Autodesk Inventor part; units mm, degrees
ref_plane "YZ Plane" through (0, 0, 0) normal (1, 0, 0) x (0, 1, 0)
ref_plane "XZ Plane" through (0, 0, 0) normal (0, 1, 0) x (-1, 0, 0)
ref_plane "XY Plane" through (0, 0, 0) normal (0, 0, 1) x (1, 0, 0)
sketch "Sketch1" plane through (0, 0, 0) normal (0, 1, 0) x (-1, 0, 0)
  line L0 (219, 0) -> (266.75, 0)
  line L1 (266.75, 0) -> (266.75, 2)
  line L2 (266.75, 2) -> (317.5, 2)
  line L3 (317.5, 2) -> (317.5, 40)
  line L4 (317.5, 40) -> (219, 40)
  line L5 (219, 40) -> (219, 0)
  line L6 (0, 0) -> (0, 40)
  line L7 (0, 40) -> (219, 40) construction
  line L8 (0, 0) -> (219, 0) construction
  line L9 (-419, 419) -> (-379, 419) construction
  line L10 (-379, 419) -> (-379, 638) construction
  line L11 (-379, 638) -> (-419, 638)
  line L12 (-419, 638) -> (-419, 419) construction
  line L13 (-379, 638) -> (-379, 736.5)
  line L14 (-379, 736.5) -> (-417, 736.5)
  line L15 (-417, 736.5) -> (-417, 685.75)
  line L16 (-417, 685.75) -> (-419, 685.75)
  line L17 (-419, 685.75) -> (-419, 638)
  dimension "d0" = 438
  dimension "d1" = 635
  dimension "d2" = 533.5
  dimension "d3" = 2
  dimension "d4" = 40
  dimension "d6" = 2
  dimension "d7" = 40
  dimension "d8" = 438
  dimension "d9" = 533.5
  dimension "d10" = 635
  dimension "d11" = 419
  dimension "d12" = 419
revolve "Revolution1" add sketch "Sketch1" angle 360 about axis through (0, 0, 0) along (0, 0, 1) contours L5 L4 L3 L2 L1 L0
revolve "Revolution2" add sketch "Sketch1" angle 360 about axis through (419, 0, 419) along (-1, 0, 0) contours L11 L17 L16 L15 L14 L13
sketch "Sketch2" plane through (0, 0, 0) normal (0, 1, 0) x (-1, 0, 0)
  line L0 (-379, 638) -> (-379, 736.5)
  line L1 (317.5, 40) -> (219, 40)
  line L2 (0, 0) -> (0, 40)
  line L3 (-419, 419) -> (-379, 419)
  arc A0 (0, 40) -> (-379, 419) centre (-379, 40) ccw
sketch "Sketch3" plane through (0, 0, 40) normal (0, 0, 1) x (1, 0, 0)
  circle A0 centre (0, 0) radius 219
  circle A1 centre (0, 0) radius 219
  circle A2 centre (0, 0) radius 230.9
  dimension "d14" = 461.8
sweep "Sweep1" add profiles "Sketch3" path "Sketch2" path curves L2 A0 L3
sketch "Sketch6" plane through (0, 0, 2) normal (0, 0, -1) x (-1, 0, 0)
  circle A0 centre (0, 0) radius 317.5
  circle A1 centre (-56.3811, -283.4469) radius 16.25
  circle A2 centre (0, 0) radius 289 construction
  line L0 (-56.3811, -283.4469) -> (0, 0) construction
  line L1 (0, 0) -> (0, -289) construction
  dimension "d20" = 11.25
  dimension "d21" = 32.5
  dimension "d22" = 578
extrude "Extrusion1" cut sketch "Sketch6" against normal up to surface (38 mm away) contours A1
pattern_circular "Circular Pattern1" count 16 over 360 about axis through (0, 0, 21) along (0, 0, -1) of "Extrusion1"
sketch "Sketch7" plane through (417, 0, 419) normal (1, 0, 0) x (0, 0, -1)
  circle A0 centre (0, 0) radius 266.75
  circle A1 centre (-56.3811, -283.4469) radius 16.25
  circle A2 centre (0, 0) radius 289 construction
  line L0 (-56.3811, -283.4469) -> (0, 0) construction
  line L1 (0, 0) -> (0, -289) construction
  dimension "d25" = 11.25
  dimension "d26" = 32.5
  dimension "d27" = 578
extrude "Extrusion2" cut sketch "Sketch7" against normal up to surface (38 mm away) contours A1
pattern_circular "Circular Pattern2" count 16 over 360 about axis through (398, 0, 419) along (-1, 0, 0) of "Extrusion2"
equation "\"d0\" = d"
equation "\"d1\" = D1"
equation "\"d2\" = D2"
equation "\"d4\" = C1"
equation "\"d7\" = C1"
equation "\"d8\" = d"
equation "\"d9\" = D2"
equation "\"d10\" = D1"
equation "\"d11\" = AA"
equation "\"d12\" = AA"
equation "\"d14\" = d + 2 * t"
equation "\"d21\" = L"
equation "\"d22\" = K1"
equation "\"d26\" = L"
equation "\"d27\" = K1"
equation "\"D1\" = 635"
equation "\"C1\" = 40"
equation "\"t\" = 11.9"
equation "\"d\" = 438"
equation "\"AA\" = 419"
equation "\"D2\" = 533.5"
equation "\"K1\" = 578"
equation "\"L\" = 32.5"
properties part number "GB/T 17185 450-PN20 \"F90E(S) RF\"" material "Steel"
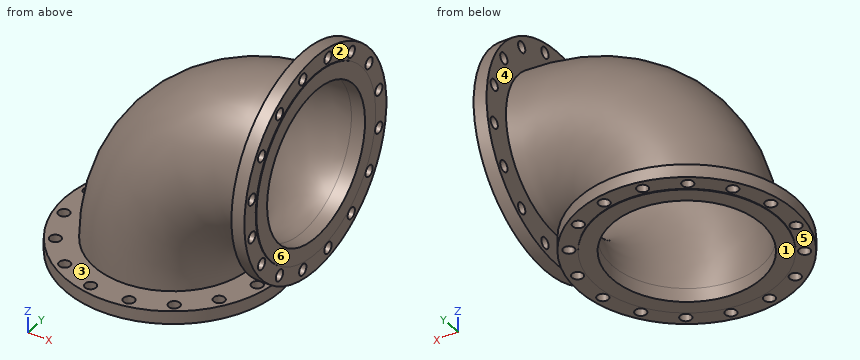
Model file for the job. Use its own axes, mm. Face numbers are marked on the shaded views. A direction names the side the tool comes from. Give positions to 0.01 mm unless a question says otherwise; leave off trailing zeros. Loops run counter-clockwise (first coordinate to the right, second up) from the corner with the lowest first, then second, coordinate; pieces in that order, holes last. Notation, with made-up numbers: (50, 45) - (100, 45) arc R28 ccw to (100, 78) - close; hole circle Ø1 at (42, -2.5). An arc over 180 degrees is marked (long way). One line per item, written item: value. Start each with the question number.
1. Probe L1, parallel to Y at x = 387, z = 409; L2, parallel to X at y = 0, z = 17; L3, parallel to Z at x = -267, y = 23. List the from-to ranges inside material, lowest first. Write a range as from..to.
2. Slice it at A-A (y = 0). List the corners of the cut face in (x, z).
3. Which spindle directions (+Z, -Z, +X, -X, +Y, -Y) get a long thin tool onto all of the face, cutting with end or side? Do the marked faces 1, 2 and 3. Say none if no direction does.
4. Pin check, flat tips, straight feed: pin 1 (19.5 mm diameter, centred on y = 160.56, z = 659.29, fed in from +X); pin 2 (19.5 mm diameter, centred on y = -160.56, z = 178.71, fed in from -X); pin 3 (6 mm diameter, centred on x = -219, y = 213.5, fed in from +Z); pin 4 (12 mm diameter, centred on y = 197.5, z = 266, fed in from -X). Stop position of each tip, or through.
5. Slice it at B-B (y = -109.5). List the corners of the cut face in (x, z), plus the area to 3 significant figures.
6. Pull direction X, two halves, no side cores. Call the marked faces 4, 5 and 6: pulls with the +X half, pulls with the -X half, needs draft (parallel to the pull), parting line crosses it, or undercut.
Solution:
1. L1: y = -317.34..-218.77, 218.77..317.34
1. L2: x = -317.5..-219, 219..317.5
1. L3: z = 2..40
2. outline: (-317.5, 2) - (-266.75, 2) - (-266.75, 0) - (-219, 0) - (-219, 40) arc R598 cw to (379, 638) - (419, 638) - (419, 685.75) - (417, 685.75) - (417, 736.5) - (379, 736.5) - (379, 649.9) arc R609.9 ccw to (-230.9, 40) - (-317.5, 40) - close; (219, 0) - (266.75, 0) - (266.75, 2) - (317.5, 2) - (317.5, 40) - (230.9, 40) arc R148.1 cw to (379, 188.1) - (379, 101.5) - (417, 101.5) - (417, 152.25) - (419, 152.25) - (419, 200) - (379, 200) arc R160 ccw to (219, 40) - close
3. face 1: -Z, +X, -X, +Y, -Y
3. face 2: +X
3. face 3: none
4. pin 1: passes through
4. pin 2: stops at x = -157.55
4. pin 3: stops at z = 40
4. pin 4: stops at x = -76.4
5. outline: (-298.02, 2) - (-243.24, 2) - (-243.24, 0) - (-189.66, 0) - (-189.66, 40) arc R568.66 cw to (379, 608.66) - (419, 608.66) - (419, 662.24) - (417, 662.24) - (417, 717.02) - (379, 717.02) - (379, 622.28) arc R582.28 ccw to (-203.28, 40) - (-298.02, 40) - close; (189.66, 0) - (243.24, 0) - (243.24, 2) - (298.02, 2) - (298.02, 40) - (203.28, 40) arc R175.72 cw to (379, 215.72) - (379, 120.98) - (417, 120.98) - (417, 175.76) - (419, 175.76) - (419, 229.34) - (379, 229.34) arc R189.34 ccw to (189.66, 40) - close
5. area: 33,100 mm^2
6. face 4: undercut
6. face 5: needs draft
6. face 6: pulls with the +X half
